Work out the finished part from the listing and answer in its coordinate system (mm). Round coordinates to 2 decimals unless told otherwise and drop trailing zeros. Loops run counter-clockwise (first coordinate to the right, second up) from the corner with the lowest first, then second, coordinate; pieces in that order, holes last. Notation, with made-up numbers: M 78.25,-34.75 L 114.25,-34.75 A32 ccw 114.25,4.25 Z; hole C -23,-39.75 d6. An arc over 180 degrees is marked long. One line per item, written item: value.
```python
from build123d import *

# Parameters (mm, degrees)
F4_R     = 10.16
F5_DEPTH = 25.4
F6_R     = 10.16
F7_DEPTH = 12.7
F8_R     = 5.08
F9_DEPTH = 25.4


with BuildPart() as f1:
    # F0 (on Front) → F1 (revolve)
    with BuildSketch(Plane.XZ):
        with BuildLine():
            Line((0, -25.4), (0, 25.4))
            ThreePointArc((0, 25.4), (-25.4, 0), (0, -25.4))
        make_face()
    revolve(axis=Axis((0, 0, 0), (0, 0, -1)))

    # F2 (on Front) → F3 (revolve)
    with BuildSketch(Plane.XZ):
        Polygon((0, 25.4), (0, 0), (76.2, 0), align=None)
    revolve(axis=Axis((38.1, 0, 0), (1, 0, 0)))

    # F4 (on Top) → F5 (cut)
    with BuildSketch(Plane.XY):
        Circle(F4_R)
    extrude(amount=-F5_DEPTH, mode=Mode.SUBTRACT)

    # F6 (on Top) → F7 (join)
    with BuildSketch(Plane.XY):
        Circle(F6_R)
    extrude(amount=-F7_DEPTH)

    # F8 (on Top) → F9 (cut)
    with BuildSketch(Plane.XY):
        with Locations((22.86, 0)):
            Circle(F8_R)
        with Locations((35.56, 0)):
            Circle(F8_R)
        with Locations((48.26, 0)):
            Circle(F8_R)
    extrude(amount=-F9_DEPTH, mode=Mode.SUBTRACT)


solid = f1.part
```
1) Find section D-D (x = 67.5). Give the vertices of the cut face in (y, z).
Check values:
outline: C 0,0 d5.8
2) Each of these flat-tipped pins is pushed along its axis until it touches: pin 1 (3 mm diameter, centred on x = 20.5, y = 0.5, fed in from -Z); pin 2 (12 mm diameter, centred on x = 8, z = -13, fed in from +Y); pin 3 (12 mm diameter, centred on x = -1, y = -13, fed in from +Z). Where does it stop, or does it pass through?
Check values:
pin 1: z = 0
pin 2: y = 23.65
pin 3: z = 24.41
3) Find the intervals of material crossed by probe 1 along X at (y, z) = (0, -18.25); probe 2 along Y at (x, z) = (44, -2.5); probe 3 along X at (y, z) = (4.5, -6), in increasing order. Write a range as from..to.
Check values:
probe 1: -17.67..-10.16, 10.16..17.78
probe 2: -10.44..-2.77, 2.77..10.44
probe 3: -24.27..20.5, 25.22..33.2, 37.92..45.9, 50.62..53.7
4) Find section A-A (x = 0). Give the vertices of the cut face in (y, z).
Check values:
outline: M -10.16,-23.28 L -10.16,-12.7 L 10.16,-12.7 L 10.16,-23.28 A25.4 ccw long Z
5) Find section B-B (z = -2). Give the number of separate pieces and of enclosed holes in the cut face, then the cut area to 3 significant figures.
Check values:
separate pieces: 1
enclosed holes: 3
area: 2,680 mm2
6) Find section C-C (x = 35.56). Give the vertices of the cut face in (y, z).
Check values:
outline: M -5.08,-12.56 L -5.08,0 L 5.08,0 L 5.08,-12.56 A13.55 ccw long Z
7) The mould has two halves that part along Y. Classify faces 1 (the face through (52.07, -2.42, 7.67)), 2 (the face through (17.785, 0.223, -9.6)): +Y half, -Y half, draft (parallel to the pull), parting line (faces both ways), or undercut.
Check values:
face 1: parting line
face 2: undercut
